from build123d import *

# Parameters (mm, degrees)
SKETCH1_W             = 100
SKETCH1_H             = 6.35
BOSS_EXTRUDE1_DEPTH   = 15.875
F_4_40_TAPPED_HOLE1_D = 2.2606
BOSS_EXTRUDE2_DEPTH   = 100
F_4_40_TAPPED_HOLE2_D = 2.2606


with BuildPart() as part:
    # Sketch1 → Boss-Extrude1 (new body)
    with BuildSketch(Plane.XY):
        with Locations((50, -3.175)):
            Rectangle(SKETCH1_W, SKETCH1_H)
    extrude(amount=BOSS_EXTRUDE1_DEPTH)

    # #4-40 Tapped Hole1 (through all)
    with Locations(Plane(origin=(0, 0, 0), x_dir=(-1, 0, 0), z_dir=(0, 0, -1))):
        with Locations((-95.72, -3.175), (-4.28, -3.175), (-34.76, -3.175), (-65.24, -3.175)):
            Hole(F_4_40_TAPPED_HOLE1_D / 2)

    # Sketch4 → Boss-Extrude2 (add, through all)
    with BuildSketch(Plane(origin=(100, 0, 0), x_dir=(0, 0, -1), z_dir=(1, 0, 0))):
        Polygon((0, 0), (-15.875, 2.51435299), (-15.875, 0), align=None)
    extrude(amount=-BOSS_EXTRUDE2_DEPTH)

    # #4-40 Tapped Hole2 (through all)
    with Locations(Plane(origin=(0, 0, 0), x_dir=(1, 0, 0), z_dir=(0, 0.987688341, -0.156434465))):
        with Locations((80.48, -13.116441936), (80.48, -2.956441936), (50, -13.116441936), (50, -2.956441936), (19.52, -13.116441936), (19.52, -2.956441936)):
            Hole(F_4_40_TAPPED_HOLE2_D / 2)


solid = part.part
The model under review builds one solid part; all positions refer to its coordinate system, in mm. Give positions to 0.01 mm unless a question says otherwise; leave off trailing zeros. Write each loop counter-clockwise with the first axis right and the second up, starting at its lowest first coordinate (ties: lowest second). Pieces come first, ordered by that corner, then holes.
1. Wall thickness on L1, parallel to Z at x = 49.5, y = -1.75 (3 decimals); L2, parallel to X at y = -1, z = 12.75; L3, parallel to X at y = -5, z = 14.5: over which ranges is each line inside the solid? List them lowest first.
2. Add section A-A, the plane x = 65.24. Write out the cut boundary in (y, z) (3 decimals).
3. Draft analysis for pull direction Y (two halves, no side actions). For faces 1 (the flat face through (49, -6.35, 8)), 2 (the flat face through (49, -3, 0)), 3 (the cylindrical face through (19, -2.16, 14.64)), state which applies: +Y half, -Y half, draft (parallel to the pull), parting line (faces both ways), or undercut.
4. Add section B-B, the plane z = 8.75. Write out the cut boundary in (x, y) (3 decimals), plus the area to 3 significant figures.
5. Add section C-C, the plane x = 26. Write out the cut boundary in (y, z) (3 decimals), plus the area to 3 significant figures.
Worked answers:
1. L1: z = 0 to 2.244, 4.297 to 12.531, 14.583 to 15.875
1. L2: x = 0 to 18.62, 20.42 to 49.1, 50.9 to 79.58, 81.38 to 100
1. L3: x = 0 to 18.47, 20.57 to 48.95, 51.05 to 79.43, 81.53 to 100
2. outline: (-6.35, 0) - (-4.305, 0) - (-4.305, 15.875) - (-6.35, 15.875) - close; (-2.045, 0) - (0, 0) - (2.514, 15.875) - (-2.045, 15.875) - close
3. face 1: -Y half
3. face 2: draft
3. face 3: undercut
4. outline: (0, -6.35) - (100, -6.35) - (100, 1.386) - (0, 1.386) - close; hole circle Ø2.261 at (4.28, -3.175); hole circle Ø2.261 at (34.76, -3.175); hole circle Ø2.261 at (65.24, -3.175); hole circle Ø2.261 at (95.72, -3.175)
4. area: 758 mm2
5. outline: (-6.35, 0) - (0, 0) - (2.514, 15.875) - (-6.35, 15.875) - close
5. area: 121 mm2
